Geometry: final body of the model. Coordinates: model frame, mm. A direction names the side the tool comes from. Give positions to 0.01 mm unless a question says otherwise; leave off trailing zeros. Order: outer loops, then holes, each group sorted by start corner. A loop starts at its lowest first (then second) coordinate and runs counter-clockwise, first axis right, second up. Notation, with made-up numbers: (86.5, 49) - (143.5, 49) arc R13 cw to (143.5, 64) - close; hole circle Ø6 at (89, -11). An arc over 180 degrees is marked (long way). One line per question, with ' | ' between items. Start each with the question number.
from build123d import *


with BuildPart() as part:
    # Sketch1 → Revolve1 (revolve)
    with BuildSketch(Plane(origin=(0, 0, 0), x_dir=(1, 0, 0), z_dir=(0, 1, 0))):
        with BuildLine():
            Line((-50, 10.152284264), (-50, 3.299492386))
            Line((-50, 3.299492386), (-59.390862944, 3.299492386))
            Line((-59.390862944, 3.299492386), (-59.390862944, 0))
            Line((-59.390862944, 0), (59.390862944, 0))
            Line((59.390862944, 0), (59.390862944, 3.299492386))
            Line((59.390862944, 3.299492386), (50, 3.299492386))
            Line((50, 3.299492386), (50, 10.152284264))
            Line((50, 10.152284264), (50, 18.484379762))
            Line((50, 18.484379762), (45.53834268, 18.484379762))
            Line((45.53834268, 18.484379762), (45.53834268, 8.678003166))
            add(Edge.make_bspline(
                [(0, 3.299492386), (14.134308112, 3.247838543), (28.352749593, 3.964388507), (42.936088831, 7.876240038), (45.53834268, 8.678003166)],
                knots=[0, 0, 0, 0, 0.749456369, 0.909412715, 0.909412715, 0.909412715, 0.909412715], degree=3))
            add(Edge.make_bspline(
                [(0, 3.299492386), (-14.134308112, 3.247838543), (-28.352749592, 3.964388507), (-42.936088831, 7.876240038), (-45.53834268, 8.678003166)],
                knots=[0, 0, 0, 0, 0.749456369, 0.909412715, 0.909412715, 0.909412715, 0.909412715], degree=3))
            Line((-45.53834268, 8.678003166), (-45.53834268, 18.484379762))
            Line((-45.53834268, 18.484379762), (-50, 18.484379762))
            Line((-50, 18.484379762), (-50, 10.152284264))
        make_face()
    revolve(axis=Axis((0, 0, 0), (-1, 0, 0)))


solid = part.part
(1) Contact query for flat-ended pins moving along their axis: P1, Ø6, axis at x = -45.5, z = 3, coming from the +Y side; P2, Ø3, axis at y = -1, z = -9, coming from the +X side; P3, Ø1.5, axis at y = -12, z = -0.5, coming from the -X side. Output: stop coordinate, or through.
(2) Access query for faces 5 (the cylindrical face through (-47.8, 18.045, 4.007)), 6 (the cylindrical face through (-54.761, -2.782, -1.774)). Directions: +Z, -Z, +X, -X, +Y, -Y. A direction counts if a zero-diameter tool reaches every point of the face in a straight line with its end or side. Return the directions, or none.
(3) Pull-direction query (X, two-part tool) for faces 1 (the flat face through (-45.538, 4, 8)), 2 (the flat face through (50, 0, 4)), 3 (the flat face through (45.538, 4, -8)), 4 (the cylindrical face through (54.63, -2.782, -1.774)); classes: +X half, -X half, draft (parallel to the pull), parting line (faces both ways), or undercut.
(4) Cut plane A-A, the plane y = -12. Return the cut outline in (x, z).
(5) Material intervals for line 1 along X through (y, z) = (12.5, 1); line 2 along Y through (x, z) = (45, -4); line 3 along Y through (x, z) = (43, -7), sorted ascending. Write a range as from..to.
Results are:
1) P1: y = 18.48 | P2: x = 50 | P3: x = -50
2) face 5: +X, -X | face 6: -X
3) face 1: undercut | face 2: +X half | face 3: undercut | face 4: draft
4) outline: (-50, -14.06) - (-45.54, -14.06) - (-45.54, 14.06) - (-50, 14.06) - close; (45.54, -14.06) - (50, -14.06) - (50, 14.06) - (45.54, 14.06) - close
5) line 1: -50..-45.54, 45.54..50 | line 2: -7.52..7.52 | line 3: -3.72..3.72
